```python
from build123d import *

# Parameters (mm, degrees)
CORTE_EXTRUS_O2_DEPTH = 170.685002284
CASCA2_T              = -1.5
ESBO_O9_R             = 3
CORTE_EXTRUS_O3_DEPTH = 168.788557539
ESBO_O10_W            = 12
ESBO_O10_H            = 39
CORTE_EXTRUS_O4_DEPTH = 1.5
ESBO_O11_W            = 8
ESBO_O11_H            = 15
CORTE_EXTRUS_O5_DEPTH = 1.5


with BuildPart() as part:
    # Esboço7 → Revolução1 (revolve)
    with BuildSketch(Plane.XY, mode=Mode.PRIVATE) as revolu_o1_sk:
        with BuildLine():
            Line((-58.672933336, 0), (-58.672933336, 5))
            ThreePointArc((-58.672933336, 5), (-22.604617679, 13.248604524), (11.327066664, 28))
            Line((11.327066664, 28), (106.327066664, 28))
            Line((106.327066664, 28), (106.327066664, 0))
            Line((106.327066664, 0), (-58.672933336, 0))
        make_face()
    revolve(revolu_o1_sk.sketch.rotate(Axis((-70.454996685, 0, 0), (1, 0, 0)), 90), axis=Axis((-70.454996685, 0, 0), (1, 0, 0)))

    # Esboço8 → Corte-extrusão2 (cut, through all)
    with BuildSketch(Plane(origin=(106.327066664, 0, 0), x_dir=(0, 0, -1), z_dir=(1, 0, 0))):
        with BuildLine():
            Line((-25.298221281, 12), (25.298221281, 12))
            ThreePointArc((25.298221281, 12), (0, 28), (-25.298221281, 12))
        make_face()
        with BuildLine():
            Line((-25.298221281, -12), (25.298221281, -12))
            ThreePointArc((25.298221281, -12), (0, -28), (-25.298221281, -12))
        make_face()
    extrude(amount=-CORTE_EXTRUS_O2_DEPTH, mode=Mode.SUBTRACT)

    # Casca2
    casca2_openings = [part.faces().sort_by_distance(p)[0] for p in [
        (106.327066664, 0, 0),
    ]]
    offset(amount=CASCA2_T, openings=casca2_openings)

    # Esboço9 → Corte-extrusão3 (cut, through all)
    with BuildSketch(Plane.ZY.offset(58.672933336)):
        Circle(ESBO_O9_R)
    extrude(amount=-CORTE_EXTRUS_O3_DEPTH, mode=Mode.SUBTRACT)

    # Esboço10 → Corte-extrusão4 (cut)
    with BuildSketch(Plane(origin=(0, 12, 0), x_dir=(1, 0, 0), z_dir=(0, 1, 0))):
        with Locations((26.327066664, 0)):
            Rectangle(ESBO_O10_W, ESBO_O10_H)
    extrude(amount=-CORTE_EXTRUS_O4_DEPTH, mode=Mode.SUBTRACT)

    # Esboço11 → Corte-extrusão5 (cut)
    with BuildSketch(Plane(origin=(0, 12, 0), x_dir=(1, 0, 0), z_dir=(0, 1, 0))):
        with Locations((91.327066664, 2.798221281)):
            Rectangle(ESBO_O11_W, ESBO_O11_H)
    extrude(amount=-CORTE_EXTRUS_O5_DEPTH, mode=Mode.SUBTRACT)


solid = part.part
```
For this review, take the finished solid that the model builds, in its own axes (mm). A direction names the side the tool comes from. Give positions to 0.01 mm unless a question says otherwise; leave off trailing zeros. Write each loop counter-clockwise with the first axis right and the second up, starting at its lowest first coordinate (ties: lowest second). Pieces come first, ordered by that corner, then holes. Notation, with made-up numbers: M 82.5,50 L 105.5,50 A17 cw 105.5,61 Z; hole C 59,-19 d8. An arc over 180 degrees is marked long. One line per item, written item: value.
1) Take a section at C-C, the plane x = -23.5. Write out the cut boundary in (y, z), then the cut area to 3 significant figures.
Results are:
outline: M -12,-4.89 A12.96 ccw 12,-4.89 L 12,4.89 A12.96 ccw -12,4.89 Z; hole M -10.5,-4.39 A11.38 ccw 10.5,-4.39 L 10.5,4.39 A11.38 ccw -10.5,4.39 Z
area: 118 mm²
2) For P1, Ø10, axis at x = -35.5, y = 6.5, coming from the +Z side; P2, Ø1.2, axis at x = 24.5, y = 11, coming from the -Z side; P3, Ø1.5, axis at x = -21, y = 1.5, coming from the -Z side; P4, Ø2, axis at y = 0, z = -0.5, coming from the +X side, all flat-tipped, find the tip position at first contact; note any pin that passes through.
Results are:
P1: stops at z = 9.99
P2: stops at z = -26
P3: stops at z = -13.97
P4: passes through
3) The part is to be moulded in two halves that separate along Z. For faces 3 (the cylindrical face through (59, 0, -28)), 4 (the flat face through (41, -12, 0)), 5 (the cylindrical face through (59, 0, 28)), 6 (the cylindrical face through (59.7, -0.2, -26.5)), say which applies: +Z half, -Z half, draft (parallel to the pull), parting line (faces both ways), or undercut.
Results are:
face 3: -Z half
face 4: draft
face 5: +Z half
face 6: undercut
4) Take a section at B-B, the plane x = 36. Write out the cut boundary in (y, z), then the cut area to 3 significant figures.
Results are:
outline: M -12,-25.3 A28 ccw 12,-25.3 L 12,25.3 A28 ccw -12,25.3 Z; hole M -10.5,-24.33 A26.5 ccw 10.5,-24.33 L 10.5,24.33 A26.5 ccw -10.5,24.33 Z
area: 218 mm²
5) For faces 1 (the flat face through (41, -10.5, 0)), 2 (the flat face through (-58.673, 3.3, 0.1)), list the 3-axis set-ups (+Z, -Z, +X, -X, +Y, -Y) from which the entire face can be reached by the end or side of a thin tool; tool diameter is ignored.
Results are:
face 1: +X
face 2: +Z, -Z, -X, +Y, -Y
6) For line 1 (Y direction, x = 82.5, z = 20.5); line 2 (Y direction, x = 91, z = -3); line 3 (Z direction, x = 16, y = -1), list the stretches that pass through material, from the lowest coordinate up. Write a range as from..to.
Results are:
line 1: y = -12..-10.5, 10.5..12
line 2: y = -12..-10.5
line 3: z = -27.98..-26.48, 26.48..27.98
7) Take a section at A-A, the plane z = 0. Write out the cut boundary in (x, y).
Results are:
outline: M -58.67,-5 A200 cw -26.54,-12 L 106.33,-12 L 106.33,-10.5 L -26.32,-10.5 A201.5 ccw -57.17,-3.69 L -57.17,-3 L -58.67,-3 Z; M -58.67,3 L -57.17,3 L -57.17,3.69 A201.5 ccw -26.32,10.5 L 20.33,10.5 L 20.33,12 L -26.54,12 A200 cw -58.67,5 Z; M 32.33,10.5 L 87.33,10.5 L 87.33,12 L 32.33,12 Z; M 95.33,10.5 L 106.33,10.5 L 106.33,12 L 95.33,12 Z
